from build123d import *

# Parameters (mm, degrees)
CROQUIS1_W              = 28.01
CROQUIS1_H              = 22.5
SALIENTE_EXTRUIR1_DEPTH = 2
CROQUIS3_R              = 2.5
SALIENTE_EXTRUIR2_DEPTH = 6
CROQUIS4_R              = 1.65
CORTAR_EXTRUIR1_DEPTH   = 5
REDONDEO1_R             = 1
REDONDEO2_R             = 1


with BuildPart() as part:
    # Croquis1 → Saliente-Extruir1 (new body)
    with BuildSketch(Plane(origin=(0, 0, 0), x_dir=(1, 0, 0), z_dir=(0, 1, 0))):
        Rectangle(CROQUIS1_W, CROQUIS1_H)
    extrude(amount=SALIENTE_EXTRUIR1_DEPTH)

    # Croquis3 → Saliente-Extruir2 (add)
    with BuildSketch(Plane(origin=(0, 2, 0), x_dir=(1, 0, 0), z_dir=(0, 1, 0))):
        with Locations(Location((-11.505, 8.75, 0), (0, 0, 90))):
            Circle(CROQUIS3_R)
        with Locations(Location((11.505, 8.75, 0), (0, 0, 90))):
            Circle(CROQUIS3_R)
        with Locations(Location((11.505, -8.75, 0), (0, 0, 270))):
            Circle(CROQUIS3_R)
        with Locations(Location((-11.505, -8.75, 0), (0, 0, 270))):
            Circle(CROQUIS3_R)
    extrude(amount=SALIENTE_EXTRUIR2_DEPTH)

    # Croquis4 → Cortar-Extruir1 (cut)
    with BuildSketch(Plane(origin=(0, 8, 0), x_dir=(1, 0, 0), z_dir=(0, 1, 0))):
        with Locations(Location((-11.505, 8.75, 0), (0, 0, 270))):
            Circle(CROQUIS4_R)
        with Locations(Location((11.505, 8.75, 0), (0, 0, 270))):
            Circle(CROQUIS4_R)
        with Locations(Location((11.505, -8.75, 0), (0, 0, 270))):
            Circle(CROQUIS4_R)
        with Locations(Location((-11.505, -8.75, 0), (0, 0, 270))):
            Circle(CROQUIS4_R)
    extrude(amount=-CORTAR_EXTRUIR1_DEPTH, mode=Mode.SUBTRACT)

    # Redondeo1
    redondeo1_edges = [part.edges().sort_by_distance(p)[0] for p in [
        (0, 0, 11.25),
        (-14.005, 0, 0),
        (0, 0, -11.25),
        (14.005, 0, 0),
    ]]
    fillet(redondeo1_edges, radius=REDONDEO1_R)

    # Redondeo2
    # the kernel refuses this fillet: 1 mm, written as the material it takes off along each edge
    with BuildSketch(Plane(origin=(-13.005, 1, 10.25), x_dir=(-1, 0, 0), z_dir=(0, 0, 1))) as redondeo2_piece_1_section:
        Polygon((0, 0), (REDONDEO2_R, 0), (REDONDEO2_R, REDONDEO2_R), (0, REDONDEO2_R), align=None)
    redondeo2_piece_1 = extrude(amount=REDONDEO2_R, mode=Mode.PRIVATE)
    redondeo2_piece_1 = redondeo2_piece_1 - Plane(origin=(-13.005, 1, 10.25), x_dir=(0.7071067811865475, 0.7071067811865475, 0), z_dir=(0, 0, 1)) * Sphere(REDONDEO2_R, mode=Mode.PRIVATE)
    add(redondeo2_piece_1, mode=Mode.SUBTRACT)
    with BuildSketch(Plane(origin=(-13.005, 1, -10.25), x_dir=(0, 0, -1), z_dir=(-1, 0, 0))) as redondeo2_piece_2_section:
        Polygon((0, 0), (REDONDEO2_R, 0), (REDONDEO2_R, REDONDEO2_R), (0, REDONDEO2_R), align=None)
    redondeo2_piece_2 = extrude(amount=REDONDEO2_R, mode=Mode.PRIVATE)
    redondeo2_piece_2 = redondeo2_piece_2 - Plane(origin=(-13.005, 1, -10.25), x_dir=(0, 0.7071067811865475, 0.7071067811865475), z_dir=(-1, 0, 0)) * Sphere(REDONDEO2_R, mode=Mode.PRIVATE)
    add(redondeo2_piece_2, mode=Mode.SUBTRACT)
    with BuildSketch(Plane(origin=(13.005, 1, 10.25), x_dir=(1, 0, 0), z_dir=(0, 0, 1))) as redondeo2_piece_3_section:
        Polygon((0, 0), (REDONDEO2_R, 0), (REDONDEO2_R, -REDONDEO2_R), (0, -REDONDEO2_R), align=None)
    redondeo2_piece_3 = extrude(amount=REDONDEO2_R, mode=Mode.PRIVATE)
    redondeo2_piece_3 = redondeo2_piece_3 - Plane(origin=(13.005, 1, 10.25), x_dir=(-0.7071067811865475, 0.7071067811865475, 0), z_dir=(0, 0, 1)) * Sphere(REDONDEO2_R, mode=Mode.PRIVATE)
    add(redondeo2_piece_3, mode=Mode.SUBTRACT)
    with BuildSketch(Plane(origin=(13.005, 1, -10.25), x_dir=(0, 0, -1), z_dir=(1, 0, 0))) as redondeo2_piece_4_section:
        Polygon((0, 0), (REDONDEO2_R, 0), (REDONDEO2_R, -REDONDEO2_R), (0, -REDONDEO2_R), align=None)
    redondeo2_piece_4 = extrude(amount=REDONDEO2_R, mode=Mode.PRIVATE)
    redondeo2_piece_4 = redondeo2_piece_4 - Plane(origin=(13.005, 1, -10.25), x_dir=(0, 0.7071067811865475, 0.7071067811865475), z_dir=(1, 0, 0)) * Sphere(REDONDEO2_R, mode=Mode.PRIVATE)
    add(redondeo2_piece_4, mode=Mode.SUBTRACT)
    with BuildSketch(Plane(origin=(14.005, 1, 11.25), x_dir=(-1, 0, 0), z_dir=(0, 1, 0)), Plane(origin=(14.005, 1, -11.25), x_dir=(0, 0, 1), z_dir=(0, 1, 0))) as redondeo2_piece_5:
        with BuildLine():
            CenterArc((REDONDEO2_R, -REDONDEO2_R), REDONDEO2_R, 90, 90)
            Line((0, -REDONDEO2_R), (0, 0))
            Line((0, 0), (REDONDEO2_R, 0))
        make_face()
    extrude(amount=3.5, mode=Mode.SUBTRACT)
    with BuildSketch(Plane(origin=(-14.005, 1, 11.25), x_dir=(1, 0, 0), z_dir=(0, 1, 0)), Plane(origin=(-14.005, 1, -11.25), x_dir=(0, 0, 1), z_dir=(0, 1, 0))) as redondeo2_piece_6:
        with BuildLine():
            CenterArc((REDONDEO2_R, REDONDEO2_R), REDONDEO2_R, 180, 90)
            Line((0, REDONDEO2_R), (0, 0))
            Line((0, 0), (REDONDEO2_R, 0))
        make_face()
    extrude(amount=3.5, mode=Mode.SUBTRACT)


solid = part.part
Verification items for the finished model (mm, model axes). A direction names the side the tool comes from. Coordinates: 2 decimals unless noted, no trailing zeros. Write each loop counter-clockwise with the first axis right and the second up, starting at its lowest first coordinate (ties: lowest second). Pieces come first, ordered by that corner, then holes. Notation, with made-up numbers: M 50.25,23 L 99.25,23 A13 cw 99.25,30 Z; hole C 69.5,43 d6. An arc over 180 degrees is marked long. Use a Markdown table: item, result.
Q1. Set-up check for faces 1 (the face through (-9.064, 4.958, -8.208)), 2 (the face through (13, 2, 11)), 3 (the face through (-13, 2, -11)): record each of +Z, -Z, +X, -X, +Y, -Y from which the full face is reachable in a straight line by a thin tool's end or side.
Reply:
| item | result |
|---|---|
| face 1 | +Y |
| face 2 | +Z, +X, +Y |
| face 3 | -Z, -X, +Y |
Q2. Thickness scan on line 1 (X direction, y = 6.75, z = 8.75) (3 decimals); line 2 (X direction, y = 5.25, z = 8); line 3 (Z direction, x = 11.25, y = 6). Record the ranges inside material, lowest first.
Reply:
| item | result |
|---|---|
| line 1 | x = -14.005 to -13.155, -9.855 to -9.005, 9.005 to 9.855, 13.155 to 14.005 |
| line 2 | x = -13.89 to -12.97, -10.04 to -9.12, 9.12 to 10.04, 12.97 to 13.89 |
| line 3 | z = -11.24 to -10.38, -7.12 to -6.26, 6.26 to 7.12, 10.38 to 11.24 |
Q3. Go/stop test with flat-tipped pins: P1, Ø1, axis at x = 12, z = -9, coming from the +Y side; P2, Ø10, axis at x = -1.5, z = 2.5, coming from the +Y side; P3, Ø1, axis at y = 4.5, z = -6, coming from the -X side. Record where each tip stops, or that it passes through.
Reply:
| item | result |
|---|---|
| P1 | stops at y = 3 |
| P2 | stops at y = 2 |
| P3 | stops at x = -12.59 |
Q4. Sectioned sample at A-A, the plane y = 5. Record the boundary of the cut face in (x, z) (3 decimals), plus the area to 3 significant figures.
Reply:
| item | result |
|---|---|
| outline | C -11.505,-8.75 d5; C -11.505,8.75 d5; C 11.505,-8.75 d5; C 11.505,8.75 d5; hole C -11.505,-8.75 d3.3; hole C -11.505,8.75 d3.3; hole C 11.505,-8.75 d3.3; hole C 11.505,8.75 d3.3 |
| area | 44.3 mm² |
Q5. Sectioned sample at C-C, the plane z = 1.25. Record the boundary of the cut face in (x, y) (3 decimals), plus the area to 3 significant figures.
Reply:
| item | result |
|---|---|
| outline | M -14.005,1 A1 ccw -13.005,0 L 13.005,0 A1 ccw 14.005,1 L 14.005,2 L -14.005,2 Z |
| area | 55.6 mm² |
Q6. Sectioned sample at B-B, the plane x = 0. Record the boundary of the cut face in (y, z), plus the area to 3 significant figures.
Reply:
| item | result |
|---|---|
| outline | M 0,-10.25 A1 ccw 1,-11.25 L 2,-11.25 L 2,11.25 L 1,11.25 A1 ccw 0,10.25 Z |
| area | 44.6 mm² |
Q7. Draft check along Z on faces 4 (the face through (0.182, 0.301, 10.965)), 5 (the face through (13.72, 0.3, -0.14)), 6 (the face through (13.72, 1.49, -10.95)), 7 (the face through (9.064, 4.958, 8.208)). Enter one of: +Z half, -Z half, draft (parallel to the pull), parting line (faces both ways), or undercut.
Reply:
| item | result |
|---|---|
| face 4 | +Z half |
| face 5 | draft |
| face 6 | -Z half |
| face 7 | undercut |
